Verification items for the finished model (mm, model axes). Face numbers are marked on the shaded views. A direction names the side the tool comes from. Coordinates: 2 decimals unless noted, no trailing zeros. Loops run counter-clockwise (first coordinate to the right, second up) from the corner with the lowest first, then second, coordinate; pieces in that order, holes last. Notation, with made-up numbers: (10, -9) - (20, -9) arc R26 ccw to (20, 15) - close; hole circle Ø5 at (19.5, -20.75). An arc over 180 degrees is marked (long way). One line per item, written item: value. Start each with the question number.
(1) Section check A-A (x = 22). Record the boundary of the cut face in (y, z).
(2) Thickness scan on probe 1 along Y at (x, z) = (148, 107); probe 2 along Y at (x, z) = (23.5, 112.5); probe 3 along X at (y, z) = (-156, 44). Record the ranges inside material, lowest first. Write a range as [from, to].
(3) Section check D-D (z = 111). Record the boundary of the cut face in (x, y).
(4) Section check C-C (y = 19.5). Record the boundary of the cut face in (x, z), plus the area to 3 significant figures.
(5) Set-up check for the marked faces 1 and 2: record each of +Z, -Z, +X, -X, +Y, -Y from which the full face is reachable in a straight line by a thin tool's end or side.
(6) Section check B-B (z = 21.5). Record the boundary of the cut face in (x, y), plus the area to 3 significant figures.
(7) Gauge pin test, flat ends, axial feed: P1, Ø1, axis at y = 10, z = 36.5, coming from the +X side; P2, Ø2, axis at x = 106, z = 4.5, coming from the -Y side. Record the tip position at first contact, or that the pin passes through.
```python
from build123d import *

# Parameters (mm, degrees)
F0_W     = 230
F0_H     = 120
F1_DEPTH = 120
F2_R     = 10
F3_DEPTH = 40
F4_W     = 484
F4_H     = 150
F5_DEPTH = 2
F6_R     = 9
F7_DEPTH = 230


with BuildPart() as f1:
    # F0 (on Top) → F1 (new body)
    with BuildSketch(Plane.XY):
        with Locations((56.06029, 41.008315)):
            Rectangle(F0_W, F0_H)
    extrude(amount=F1_DEPTH)

    # F2 (on face) → F3 (join)
    with BuildSketch(Plane.YZ.offset(171.06029)):
        with Locations((41.008315, 60)):
            Circle(F2_R)
    extrude(amount=F3_DEPTH)

    # F4 (on face) → F5 (join)
    with BuildSketch(Plane.YZ.offset(171.06029)):
        with Locations((41.008315, 45)):
            Rectangle(F4_W, F4_H)
    extrude(amount=F5_DEPTH)

    # F6 (on face) → F7 (join)
    with BuildSketch(Plane(origin=(171.06029, 0, 0), x_dir=(0, -1, 0), z_dir=(-1, 0, 0))):
        with Locations((180.991685, 111)):
            Circle(F6_R)
        with Locations((-263.008315, 111)):
            Circle(F6_R)
    extrude(amount=F7_DEPTH)


solid = f1.part
```
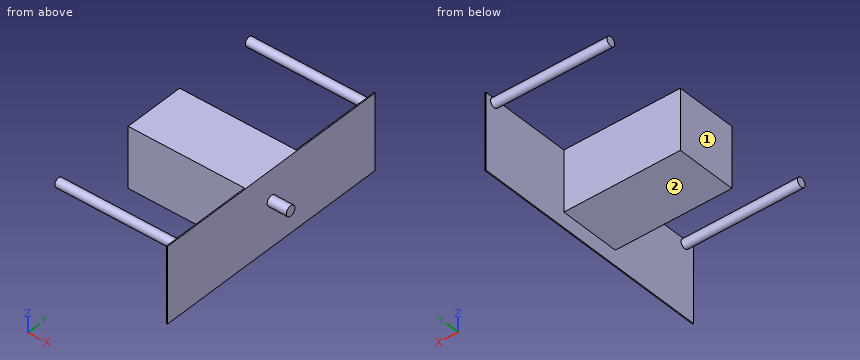
Responses:
1. outline: circle Ø18 at (-180.99, 111); (-18.99, 0) - (101.01, 0) - (101.01, 120) - (-18.99, 120) - close; circle Ø18 at (263.01, 111)
2. probe 1: y = [-189.05, -172.93], [-18.99, 101.01], [254.95, 271.07]
2. probe 2: y = [-189.87, -172.12], [-18.99, 101.01], [254.13, 271.88]
2. probe 3: x = [171.06, 173.06]
3. outline: (-58.94, -189.99) - (171.06, -189.99) - (171.06, -200.99) - (173.06, -200.99) - (173.06, 283.01) - (171.06, 283.01) - (171.06, 272.01) - (-58.94, 272.01) - (-58.94, 254.01) - (171.06, 254.01) - (171.06, 101.01) - (-58.94, 101.01) - (-58.94, -18.99) - (171.06, -18.99) - (171.06, -171.99) - (-58.94, -171.99) - close
4. outline: (-58.94, 0) - (171.06, 0) - (171.06, -30) - (173.06, -30) - (173.06, 120) - (-58.94, 120) - close
4. area: 27,900 mm²
5. face 1: +Z, -Z, -X, +Y, -Y
5. face 2: -Z, -X, +Y, -Y
6. outline: (-58.94, -18.99) - (171.06, -18.99) - (171.06, -200.99) - (173.06, -200.99) - (173.06, 283.01) - (171.06, 283.01) - (171.06, 101.01) - (-58.94, 101.01) - close
6. area: 28,600 mm²
7. P1: stops at x = 173.06
7. P2: stops at y = -18.99
